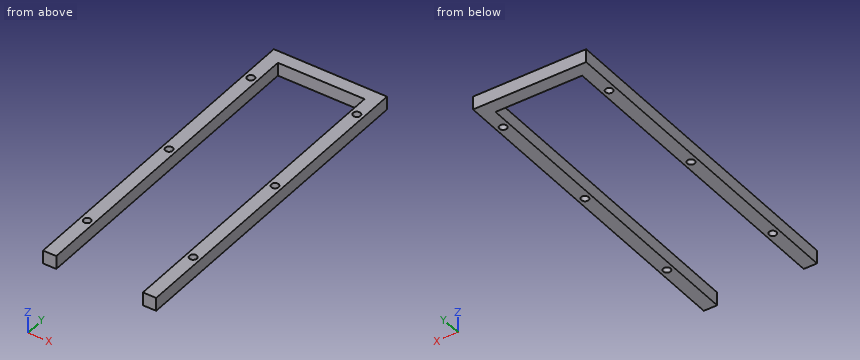
Autodesk Inventor part; units mm, degrees
ref_plane "YZ Plane" through (0, 0, 0) normal (1, 0, 0) x (0, 1, 0)
ref_plane "XZ Plane" through (0, 0, 0) normal (0, 1, 0) x (-1, 0, 0)
ref_plane "XY Plane" through (0, 0, 0) normal (0, 0, 1) x (1, 0, 0)
sketch "Esboço1" plane through (0, 0, 0) normal (0, 1, 0) x (-1, 0, 0)
  line L0 (0, 0) -> (0, -5.4)
  line L1 (0, -5.4) -> (5.4, -5.4)
  line L2 (5.4, -5.4) -> (5.4, 0)
  line L3 (5.4, 0) -> (0, 0)
  line L4 (40.622, 0) -> (40.622, -5.4)
  line L5 (40.622, -5.4) -> (46.022, -5.4)
  line L6 (46.022, -5.4) -> (46.022, 0)
  line L7 (46.022, 0) -> (40.622, 0)
  line L8 (40.622, 0) -> (5.4, 0)
  line L9 (5.4, -5.4) -> (40.622, -5.4)
  point P0 (0, -2.7)
  point P1 (5.4, -2.7)
  point P2 (40.622, -2.7)
  point P3 (46.022, -2.7)
  point P4 (43.322, -5.4)
  point P5 (2.7, -5.4)
  point P6 (43.322, 0)
  point P7 (2.7, 0)
  point P8 (0, 0)
  dimension "d29" = 35.222
  dimension "d30" = 5.4
extrude "Extrusão1" add sketch "Esboço1" against normal blind 130 contours L3 L2 L1 L0 | L7 L6 L5 L4
extrude "Extrusão4" add sketch "Esboço1" along normal blind 5.4
sketch "Esboço5" plane through (-40.622, 0, 0) normal (0, 0, 1) x (1, 0, 0)
  circle A0 centre (37.922, -104.396) radius 1.5
  circle A1 centre (37.922, -56.396) radius 1.5
  circle A2 centre (37.922, -8.397) radius 1.5
  circle A3 centre (-2.7, -107.95) radius 1.5
  circle A4 centre (-2.7, -59.95) radius 1.5
  circle A5 centre (-2.7, -11.951) radius 1.5
  line L0 (40.622, -130) -> (35.222, -130)
  line L1 (0, -130) -> (-5.4, -130)
  line L2 (37.7913, -105.8903) -> (103.7232, -105.8903) construction
  line L3 (38.0527, -57.8903) -> (-2.5693, -61.4443)
  line L4 (38.0527, -9.8913) -> (-2.5693, -13.4453)
  line L5 (-2.5693, -109.4443) -> (38.0527, -105.8903)
  point P0 (40.622, 0)
  point P1 (37.922, -130)
  point P2 (-2.7, -130)
  dimension "d33" = 3
  dimension "d34" = 3
  dimension "d36" = 3
  dimension "d38" = 3
  dimension "d40" = 3
  dimension "d42" = 3
  dimension "d44" = 25.604
  dimension "d45" = 48
  dimension "d46" = 47.999
  dimension "d52" = 5
extrude "Extrusão5" cut sketch "Esboço5" against normal through all
equation "\"d29\" = Largura_trilhos"
equation "\"d33\" = Parafuso"
equation "\"d34\" = d35"
equation "\"d36\" = d37"
equation "\"d38\" = d39"
equation "\"d40\" = d41"
equation "\"d42\" = d43"
equation "\"Largura_trilhos\" = 35.222"
equation "\"Parafuso\" = 3"
equation "\"d11\" = 3"
equation "\"d13\" = 3"
equation "\"d15\" = 3"
equation "\"d17\" = 3"
equation "\"d19\" = 3"
equation "\"d35\" = 3"
equation "\"d37\" = 3"
equation "\"d39\" = 3"
equation "\"d41\" = 3"
equation "\"d43\" = 3"
properties part number "Sustentação Trilhos fixos" material "Plástico PET"
Can you work these out from the model? Positions are in its coordinate system, mm. Coordinates: 2 decimals unless noted, no trailing zeros. Loops run counter-clockwise (first coordinate to the right, second up) from the corner with the lowest first, then second, coordinate; pieces in that order, holes last.
1) For pin 1 (2.5 mm diameter, centred on x = -2.7, y = -104.396, fed in from +Z), with a flat end and sliding along its axis, tell me the tip position at first contact or that it passes through.
2) Imagine slicing it at B-B on x = -2.7. List the corners of the cut face in (y, z) for me, plus the area to 3 significant figures.
3) Imagine slicing it at C-C on y = -64. List the corners of the cut face in (x, z) for me, plus the area to 3 significant figures.
4) Imagine slicing it at A-A on y = -107.95. List the corners of the cut face in (x, z) for me, plus the area to 3 significant figures.
5) Imagine slicing it at D-D on z = -4.5. List the corners of the cut face in (x, y) for me.
6) I need wall thicknesses on probe 1 along Y at (x, z) = (-2.7, -2.6); probe 2 along X at (y, z) = (-13, -2.05); probe 3 along X at (y, z) = (-75, -3.7). Which ranges of each line are inside material? Lowest first, please.
Completed:
1. pin 1: passes through
2. outline: (-130, -5.4) - (-105.9, -5.4) - (-105.9, 0) - (-130, 0) - close; (-102.9, -5.4) - (-57.9, -5.4) - (-57.9, 0) - (-102.9, 0) - close; (-54.9, -5.4) - (-9.9, -5.4) - (-9.9, 0) - (-54.9, 0) - close; (-6.9, -5.4) - (5.4, -5.4) - (5.4, 0) - (-6.9, 0) - close
2. area: 683 mm2
3. outline: (-46.02, -5.4) - (-40.62, -5.4) - (-40.62, 0) - (-46.02, 0) - close; (-5.4, -5.4) - (0, -5.4) - (0, 0) - (-5.4, 0) - close
3. area: 58.3 mm2
4. outline: (-46.02, -5.4) - (-44.82, -5.4) - (-44.82, 0) - (-46.02, 0) - close; (-41.82, -5.4) - (-40.62, -5.4) - (-40.62, 0) - (-41.82, 0) - close; (-5.4, -5.4) - (0, -5.4) - (0, 0) - (-5.4, 0) - close
4. area: 42.1 mm2
5. outline: (-46.02, -130) - (-40.62, -130) - (-40.62, 0) - (-5.4, 0) - (-5.4, -130) - (0, -130) - (0, 5.4) - (-46.02, 5.4) - close; hole circle Ø3 at (-43.32, -107.95); hole circle Ø3 at (-43.32, -59.95); hole circle Ø3 at (-43.32, -11.95); hole circle Ø3 at (-2.7, -104.4); hole circle Ø3 at (-2.7, -56.4); hole circle Ø3 at (-2.7, -8.4)
6. probe 1: y = -130 to -105.9, -102.9 to -57.9, -54.9 to -9.9, -6.9 to 5.4
6. probe 2: x = -46.02 to -44.39, -42.25 to -40.62, -5.4 to 0
6. probe 3: x = -46.02 to -40.62, -5.4 to 0
